from build123d import *

# Parameters (mm, degrees)
F0_R     = 2
F1_DEPTH = 3


with BuildPart() as f1:
    # F0 (on Front) → F1 (new body)
    with BuildSketch(Plane.XZ):
        Polygon((-116.36717, 91.362698), (-116.36717, 61.206273), (-108.296373, 50.529602), (-108.296373, 70.491589), (-105.836282, 74.723937), (-102.795032, 70.700737), (-102.795032, 50.529602), (-96.265585, 50.529602), (-96.265585, 70.393569), (-93.008241, 74.651143), (-89.701266, 70.393569), (-89.701266, 50.529602), (-83.244497, 50.529602), (-83.244497, 70.423895), (-79.906239, 73.922077), (-77.148117, 70.423895), (-77.148117, 50.529602), (-71.271746, 50.529602), (-71.271746, 69.549546), (-67.90149, 73.764265), (-64.586512, 69.549546), (-64.586512, 50.529602), (-58.640746, 50.529602), (-58.640746, 69.340751), (-54.856984, 74.066021), (-51.358108, 69.340751), (-51.358108, 50.529602), (-46.37086, 50.529602), (-46.37086, 68.703967), (-42.394505, 73.879614), (-38.753841, 68.703967), (-38.753841, 50.529602), (-32.736491, 50.529602), (-32.736491, 69.565687), (-29.575566, 74.61762), (-26.222558, 69.565687), (-26.222558, 50.529602), (-21.325707, 50.529602), (-21.325707, 70.393569), (-18.979074, 74.651143), (-15.930735, 70.393569), (-15.930735, 50.529602), (-11.662976, 50.529602), (-11.662976, 70.393569), (-9.12501, 74.723019), (-6.402003, 70.393569), (-6.402003, 50.529602), (-1.288212, 50.529602), (-1.288212, 70.393569), (1.289989, 74.651143), (3.614716, 70.393569), (3.614716, 50.529602), (6.625234, 50.529602), (6.625234, 70.468216), (8.86461, 74.424437), (11.610716, 70.696345), (11.610716, 50.529602), (15.495674, 50.529602), (21.029814, 63.529602), (21.029814, 91.2588), (13.958036, 91.197406), (-7.926733, 91.007412), (-109.232884, 91.362698), align=None)
        with BuildLine():
            ThreePointArc((-86.268887, 134.798962), (-104.59103, 116.697095), (-109.232884, 91.362698))
            Line((-109.232884, 91.362698), (-7.926733, 91.007412))
            Line((-7.926733, 91.007412), (13.958036, 91.197406))
            ThreePointArc((13.958036, 91.197406), (8.519054, 116.737455), (-10.339861, 134.798962))
            Line((-10.339861, 134.798962), (-14.25776, 134.798962))
            Line((-14.25776, 134.798962), (-14.25776, 137.639998))
            Line((-14.25776, 137.639998), (-17.807812, 137.639998))
            ThreePointArc((-17.807812, 137.639998), (-30.698392, 140.973244), (-43.974803, 141.980461))
            ThreePointArc((-43.974803, 141.980461), (-61.091751, 141.192299), (-77.854575, 137.639998))
            Line((-77.854575, 137.639998), (-81.178934, 137.639998))
            Line((-81.178934, 137.639998), (-81.178934, 134.798962))
            Line((-81.178934, 134.798962), (-86.268887, 134.798962))
        make_face()
        with Locations((-46.382562, 136.033968)):
            Circle(F0_R, mode=Mode.SUBTRACT)
        Polygon((-127.604582, 61.206273), (-127.604582, 3.529602), (27.042171, 3.529602), (27.042171, 63.529602), (21.029814, 63.529602), (15.495674, 50.529602), (11.610716, 50.529602), (6.625234, 50.529602), (3.614716, 50.529602), (-1.288212, 50.529602), (-6.402003, 50.529602), (-11.662976, 50.529602), (-15.930735, 50.529602), (-21.325707, 50.529602), (-26.222558, 50.529602), (-32.736491, 50.529602), (-38.753841, 50.529602), (-46.37086, 50.529602), (-51.358108, 50.529602), (-58.640746, 50.529602), (-64.586512, 50.529602), (-71.271746, 50.529602), (-77.148117, 50.529602), (-83.244497, 50.529602), (-89.701266, 50.529602), (-96.265585, 50.529602), (-102.795032, 50.529602), (-108.296373, 50.529602), (-116.36717, 61.206273), align=None)
        Polygon((-153.489637, -9.072431), (-153.489637, -19.268759), (57.278608, -19.268759), (57.278608, -9.072431), (41.525324, -9.072431), (-139.909211, -9.072431), align=None)
        Polygon((-139.909211, 3.529602), (-139.909211, -9.072431), (41.525324, -9.072431), (41.525324, 3.529602), (27.042171, 3.529602), (-127.604582, 3.529602), align=None)
        Polygon((-153.489637, -19.268759), (-179.380361, -19.268759), (-179.380361, -49.268759), (79.836207, -49.268759), (79.836207, -19.268759), (57.278608, -19.268759), align=None)
        with Locations((-163.380361, -34.268759)):
            Circle(F0_R, mode=Mode.SUBTRACT)
        with Locations((66.836207, -34.268759)):
            Circle(F0_R, mode=Mode.SUBTRACT)
    extrude(amount=F1_DEPTH)


solid = f1.part
Work out the finished part from the listing and answer in its coordinate system (mm). Round coordinates to 2 decimals unless told otherwise and drop trailing zeros. Loops run counter-clockwise (first coordinate to the right, second up) from the corner with the lowest first, then second, coordinate; pieces in that order, holes last. Notation, with made-up numbers: (78, 33) - (100, 33) arc R37 ccw to (100, 70) - close; hole circle Ø10 at (11, 40.5). An arc over 180 degrees is marked (long way). Use one line per item in the form item = value. Start each with the question number.
(1) Find section A-A on x = 36.5. Determine the outline of the cut face in (y, z).
(2) Flat-ended cylindrical pins translate along their axes: P1, Ø0.9, axis at y = -1.5, z = -12, coming from the -X side; P2, Ø0.9, axis at y = -2, z = 57.5, coming from the -X side; P3, Ø1.5, axis at y = -1.5, z = 59.5, coming from the +X side. Find the tip coordinate at first contact, or state that the pin passes through.
(3) Find section C-C on y = -1. Give the number of separate pieces and of enclosed holes in the cut face, and give its area (3 significant figures).
(4) Find section B-B on z = -13. Determine the outline of the cut face in (x, y), and give its area (3 significant figures).
(5) Consider line 1 (Z direction, x = 22.5, y = -0.2); line 2 (Z direction, x = 40, y = -1.85); line 3 (X direction, y = -0.2, z = 1). Determine where each line is inside the solid, lowest interval first.
Answer list:
q1.outline = (-3, -49.27) - (0, -49.27) - (0, 3.53) - (-3, 3.53) - close
q2.P1 = -153.49
q2.P2 = -127.6
q2.P3 = 27.04
q3.separate_pieces = 1
q3.enclosed_holes = 14
q3.area = 29,000 mm^2
q4.outline = (-153.49, -3) - (57.28, -3) - (57.28, 0) - (-153.49, 0) - close
q4.area = 632 mm^2
q5.line_1 = -49.27 to 63.53
q5.line_2 = -49.27 to 3.53
q5.line_3 = -139.91 to 41.53
